```python
from build123d import *

# Parameters (mm, degrees)
BOX001_W       = 10
BOX001_H       = 10
BOX001_DEPTH   = 8
CYLINDER_R     = 2.5
CYLINDER_DEPTH = 5
SKETCH_R       = 3
EXTRUDE_DEPTH  = 14
BOX_W          = 16
BOX_H          = 16
BOX_DEPTH      = 10


with BuildPart() as cube001:
    # Box001 → Box001 (new body)
    with BuildSketch(Plane(origin=(-5, -5, 0), x_dir=(1, 0, 0), z_dir=(0, 0, 1))):
        with Locations((5, 5)):
            Rectangle(BOX001_W, BOX001_H)
    extrude(amount=BOX001_DEPTH)


with BuildPart() as cylinder:
    # Cylinder → Cylinder (new body)
    with BuildSketch(Plane.XY.offset(10)):
        Circle(CYLINDER_R)
    extrude(amount=CYLINDER_DEPTH)


with BuildPart() as extrude_body:
    # Sketch (on Cylinder) → Extrude (new body)
    with BuildSketch(Plane(origin=(0, 0, 10), x_dir=(1, 0, 0), z_dir=(0, -1, 0))):
        with Locations((0, 7)):
            Circle(SKETCH_R)
    extrude(amount=EXTRUDE_DEPTH)


with BuildPart() as extrude_body_1:
    # Extrude placement: moved
    add(extrude_body.part.moved(Location((0, 7, 0))))


with BuildPart() as cut:
    # Box → Box (new body)
    with BuildSketch(Plane(origin=(-8, -8, 0), x_dir=(1, 0, 0), z_dir=(0, 0, 1))):
        with Locations((8, 8)):
            Rectangle(BOX_W, BOX_H)
    extrude(amount=BOX_DEPTH)

    # Fusion: union Cylinder, Extrude body
    add(cylinder.part)
    add(extrude_body_1.part)

    # Cut: cut Cube001
    add(cube001.part, mode=Mode.SUBTRACT)


solid = cut.part
```
Input: part model. Units: mm. Frame: model coordinates. A direction names the side the tool comes from. Give positions to 0.01 mm unless a question says otherwise; leave off trailing zeros. Loops run counter-clockwise (first coordinate to the right, second up) from the corner with the lowest first, then second, coordinate; pieces in that order, holes last.
1) Section query A-A on y = 3.25. Return the cut outline in (x, z).
A:
outline: (-8, 0) - (-5, 0) - (-5, 8) - (5, 8) - (5, 0) - (8, 0) - (8, 10) - (-8, 10) - close; circle Ø6 at (0, 17)
2) Reachability of faces 1 (the flat face through (0, 7, 17)), 2 (the flat face through (0, -7, 17)), 3 (the flat face through (0, 0, 8)), 4 (the flat face through (-2, 2, 10)) from +Z, -Z, +X, -X, +Y, -Y: full face, straight path, thin tool, end or side. Return the list, or none.
A:
face 1: +Z, +X, -X, +Y
face 2: +Z, +X, -X, -Y
face 3: -Z
face 4: none
3) Section query D-D on y = 0. Return the cut outline in (x, z).
A:
outline: (-8, 0) - (-5, 0) - (-5, 8) - (5, 8) - (5, 0) - (8, 0) - (8, 10) - (2.5, 10) - (2.5, 15) - (2.24, 15) arc R3 ccw (long way) to (-2.24, 15) - (-2.5, 15) - (-2.5, 10) - (-8, 10) - close
4) Line query: L1, parallel to X at y = -3.5, z = 4.25; L2, parallel to Z at x = 3.5, y = -3.5. Output: solid intervals per line, ascending.
A:
L1: x = -8 to -5, 5 to 8
L2: z = 8 to 10
5) Contact query for flat-ended pins moving along their axis: pin 1 (5 mm diameter, centred on x = 1, z = 17, fed in from +Y); pin 2 (6 mm diameter, centred on x = -5, z = 10.5, fed in from +Y); pin 3 (3 mm diameter, centred on x = -1.5, z = 17.5, fed in from -Y); pin 4 (1.5 mm diameter, centred on x = 1.5, y = -1, fed in from -Z). Output: stop coordinate, or through.
A:
pin 1: stops at y = 7
pin 2: stops at y = 8
pin 3: stops at y = -7
pin 4: stops at z = 8
6) Section query B-B on z = 4. Return the cut outline in (x, y), and give its area (3 significant figures).
A:
outline: (-8, -8) - (8, -8) - (8, 8) - (-8, 8) - close; hole (-5, -5) - (5, -5) - (5, 5) - (-5, 5) - close
area: 156 mm2
7) Section query C-C on x = 0. Return the cut outline in (y, z).
A:
outline: (-8, 0) - (-5, 0) - (-5, 8) - (5, 8) - (5, 0) - (8, 0) - (8, 10) - (2.5, 10) - (2.5, 14) - (7, 14) - (7, 20) - (-7, 20) - (-7, 14) - (-2.5, 14) - (-2.5, 10) - (-8, 10) - close
8) Mould query, pull axis X, two halves, no side actions, for faces 5 (the flat face through (0, -8, 5)), 6 (the flat face through (0, -5, 4)), 7 (the cylindrical face through (1.15, -2.22, 12.47)). Classes: released by +X, released by -X, zero draft, split by the parting line, or undercut.
A:
face 5: zero draft
face 6: undercut
face 7: split by the parting line
